Input: part model. Units: mm. Frame: model coordinates. A direction names the side the tool comes from. Coordinates: 2 decimals unless noted, no trailing zeros. Write each loop counter-clockwise with the first axis right and the second up, starting at its lowest first coordinate (ties: lowest second). Pieces come first, ordered by that corner, then holes. Notation, with made-up numbers: (-28.75, 9) -> (5.25, 9) arc R12 ccw to (5.25, 27) -> close; hole circle Ø6 at (32, 6.5). An arc over 180 degrees is marked (long way). Use one line per item in the form item = value. Start each with the question number.
(1) Cut plane B-B on x = 21.5. Return the cut outline in (y, z).
(2) Pull-direction query (X, two-part tool) for faces 1 (the face through (26.797, 12, 6)), 2 (the face through (67, 8, 10.2)), 3 (the face through (60.635, 7.672, 12.284)), 4 (the face through (63, 5.08, 5)); classes: released by +X, released by -X, zero draft, split by the parting line, or undercut.
(3) First-contact query: pin 1 (5.5 mm diameter, centred on y = 3.5, z = 4.5, fed in from -X); pin 2 (1.5 mm diameter, centred on y = 3, z = 3.5, fed in from -X); pin 3 (4 mm diameter, centred on x = 22.606, z = 6.35, fed in from -Y); pin 4 (1.5 mm diameter, centred on y = 1.5, z = 5.5, fed in from +X). Flat tips, straight axial feed; report the tip coordinate or a pass-through.
(4) Cut plane A-A on y = 3.25. Return the cut outline in (x, z).
(5) Ray query, line 1 along X through (y, z) = (4.5, 2); line 2 along X through (y, z) = (7.55, 6.35); line 3 along Z through (x, y) = (22.5, 10.5). Return the intervals inside material, ascending.
(6) Set-up query: faces 5 (the face through (66.802, 3, 5)), 6 (the face through (56.896, 3, 6)), 7 (the face through (68.41, 0.93, 8.25)). Return all of +Z, -Z, +X, -X, +Y, -Y with unobstructed straight access to the full face (end or side cutting, diameter ignored); none if empty.
(7) Cut plane D-D on x = 40.5. Return the cut outline in (y, z).
(8) Cut plane C-C on z = 8.75. Return the cut outline in (x, y).
```python
from build123d import *

# Parameters (mm, degrees)
CROQUIS1_W              = 74.93
CROQUIS1_H              = 12.7
SALIENTE_EXTRUIR1_DEPTH = 12.7
CROQUIS2_W              = 26.797
CROQUIS2_H              = 1.6764
CROQUIS2_W_2            = 6.731
CROQUIS2_H_2            = 5.08
CROQUIS2_W_3            = 56.896
CROQUIS2_W_4            = 4.953
CORTAR_EXTRUIR1_DEPTH   = 78.052481466
TALADRO_ROSCADO_8_321_D = 3.4544
CORTAR_EXTRUIR2_DEPTH   = 78.052481466
CORTAR_EXTRUIR3_DEPTH   = 78.052481466


with BuildPart() as part:
    # Croquis1 → Saliente-Extruir1 (new body)
    with BuildSketch(Plane(origin=(0, 0, 0), x_dir=(1, 0, 0), z_dir=(0, 1, 0))):
        with Locations((37.465, -6.35)):
            Rectangle(CROQUIS1_W, CROQUIS1_H)
    extrude(amount=SALIENTE_EXTRUIR1_DEPTH)

    # Croquis2 → Cortar-Extruir1 (cut, through all)
    with BuildSketch(Plane.XY.offset(12.7)):
        with Locations((13.3985, 11.8618)):
            Rectangle(CROQUIS2_W, CROQUIS2_H)
        with Locations((63.4365, 2.54)):
            Rectangle(CROQUIS2_W_2, CROQUIS2_H_2)
        with Locations((28.448, 2.54)):
            Rectangle(CROQUIS2_W_3, CROQUIS2_H_2)
        with Locations((72.4535, 2.54)):
            Rectangle(CROQUIS2_W_4, CROQUIS2_H_2)
    extrude(amount=-CORTAR_EXTRUIR1_DEPTH, mode=Mode.SUBTRACT)

    # Taladro roscado #8-321 (through all)
    with Locations(Plane(origin=(0, 5.08, 0), x_dir=(-1, 0, 0), z_dir=(0, -1, 0))):
        with Locations((-4.318, -6.35), (-13.462, -6.35), (-22.606, -6.35)):
            Hole(TALADRO_ROSCADO_8_321_D / 2)

    # Croquis6 → Cortar-Extruir2 (cut, through all)
    with BuildSketch(Plane.XZ):
        with BuildLine():
            Line((68.58, 10.2), (63.4238, 10.2))
            ThreePointArc((63.4238, 10.2), (61.191404448, 12.04078202), (58.374047531, 12.7))
            Line((58.374047531, 12.7), (74.93, 12.7))
            Line((74.93, 12.7), (74.93, 3.85))
            ThreePointArc((74.93, 3.85), (73.070128061, 8.340128061), (68.58, 10.2))
        make_face()
    extrude(amount=-CORTAR_EXTRUIR2_DEPTH, mode=Mode.SUBTRACT)

    # Croquis7 → Cortar-Extruir3 (cut, through all)
    with BuildSketch(Plane(origin=(74.93, 0, 0), x_dir=(0, 0, -1), z_dir=(1, 0, 0))):
        Polygon((-2.3622, 0), (-6.35, 1.778), (-10.3378, 0), align=None)
    extrude(amount=-CORTAR_EXTRUIR3_DEPTH, mode=Mode.SUBTRACT)


solid = part.part
```
Values:
q1.outline = (5.08, 0) -> (11.02, 0) -> (11.02, 5.02) -> (5.08, 5.02) -> close; (5.08, 7.68) -> (11.02, 7.68) -> (11.02, 12.7) -> (5.08, 12.7) -> close
q2.face_1 = released by -X
q2.face_2 = zero draft
q2.face_3 = released by +X
q2.face_4 = undercut
q3.pin_1 = 0
q3.pin_2 = 56.9
q3.pin_3 = 5.08
q3.pin_4 = 69.98
q4.outline = (56.9, 0) -> (60.07, 0) -> (60.07, 12.47) arc R6.35 ccw to (58.37, 12.7) -> (56.9, 12.7) -> close; (66.8, 0) -> (69.98, 0) -> (69.98, 10.04) arc R6.35 ccw to (68.58, 10.2) -> (66.8, 10.2) -> close
q5.line_1 = 56.9 to 60.07, 66.8 to 69.98
q5.line_2 = 0 to 2.59, 6.05 to 11.73, 15.19 to 20.88, 24.33 to 74.42
q5.line_3 = 0 to 4.63, 8.07 to 12.7
q6.face_5 = +Z, -Z, -Y
q6.face_6 = +Z, -Z, -X, -Y
q6.face_7 = +X, -X, -Y
q7.outline = (5.08, 0) -> (12.7, 0) -> (12.7, 12.7) -> (5.08, 12.7) -> close
q8.outline = (0, 5.08) -> (56.9, 5.08) -> (56.9, 0.71) -> (60.07, 0.71) -> (60.07, 5.08) -> (66.8, 5.08) -> (66.8, 0.71) -> (69.98, 0.71) -> (69.98, 5.08) -> (72.62, 5.08) -> (72.62, 12.7) -> (26.8, 12.7) -> (26.8, 11.02) -> (0, 11.02) -> close
